Here's how the part is built. I have some questions about the finished solid (model axes, mm). A direction names the side the tool comes from. Coordinates: 2 decimals unless noted, no trailing zeros. Loops run counter-clockwise (first coordinate to the right, second up) from the corner with the lowest first, then second, coordinate; pieces in that order, holes last. Notation, with made-up numbers: M 5.5,33.25 L 38.5,33.25 A13 ccw 38.5,39.25 Z; hole C -27,12 d3. An arc over 180 degrees is marked long. Use CSV: the item, a comma, the result in double quotes. Start each with the question number.
Q1. If we section it at B-B (z = 5.25): Please give me the cut outline in (x, y).
Q2. Please list where these lines run through material, in increasing order: probe 1 along Y at (x, z) = (0, 12.5); probe 2 along Y at (x, z) = (1.5, 10.5). Write a range as [from, to].
Q3. If we section it at C-C (x = 14): Please give me the cut outline in (y, z).
Q4. Which directions (+Z, -Z, +X, -X, +Y, -Y) give clear straight access to the entire face, cutting with the end or side of a thin tool? Please do faces 1 (the flat face through (-14, 0, 18)), 2 (the flat face through (1.204, 14, 19)), 3 (the flat face through (-11, 12, 5.94)), 4 (the flat face through (13, -9, 3)).
Q5. For pin 1 Ø8 at (y, z) = (10, 14.5) entering from +X; pin 2 Ø4 at (x, y) = (-5, 12.5) entering from -Z; pin 3 Ø0.8 at (y, z) = (-14, 19) entering from +X; pin 4 Ø2.5 at (x, z) = (13.5, 2) entering from -Y, each with a flat end and sliding along its axis, tell me the tip position at first contact or that it passes through.
Q6. If we section it at A-A (y = 0): Please give me the cut outline in (x, z), and give its area (3 significant figures).
Q7. If we mould it in two halves opening along X, with no side actions, what happens to faces 5 (the flat face through (0, 14, 18)), 6 (the flat face through (0, -16, 0)), 7 (the flat face through (1.204, -14, 19))? For each: +X half, -X half, draft (parallel to the pull), parting line (faces both ways), or undercut.
Q8. If we section it at D-D (x = 0): Please give me the cut outline in (y, z).
from build123d import *

# Parameters (mm, degrees)
F0_R     = 17
F0_R_2   = 15
F1_DEPTH = 20
F3_DEPTH = 25
F5_DEPTH = 2
F7_DEPTH = 2


with BuildPart() as f1:
    # F0 (on Top) → F1 (new body)
    with BuildSketch(Plane.XY):
        Circle(F0_R)
        Circle(F0_R_2, mode=Mode.SUBTRACT)
    extrude(amount=F1_DEPTH)

    # F2 (on Right) → F3 (cut, symmetric)
    with BuildSketch(Plane.YZ):
        Polygon((-9, 5.94), (-9, -6.120001), (9, -5.76), (9, 5.94), (14, 5.94), (14, 9.000001), (-14, 9.000001), (-14, 5.94), align=None)
    extrude(amount=F3_DEPTH, both=True, mode=Mode.SUBTRACT)

    # F4 (on face) → F5 (join)
    with BuildSketch(Plane.XY.offset(20)):
        with BuildLine():
            ThreePointArc((-14.831288, -2.243409), (-14.998609, -0.204311), (-14.886893, 1.838588))
            Line((-14.886893, 1.838588), (-16.424584, 1.838588))
            Line((-16.424584, 1.838588), (-16.424584, -2.243409))
            Line((-16.424584, -2.243409), (-14.831288, -2.243409))
        make_face()
        with BuildLine():
            Line((-12.919951, -2.243409), (-12.919951, 1.838588))
            Line((-12.919951, 1.838588), (-14.886893, 1.838588))
            ThreePointArc((-14.886893, 1.838588), (-14.998609, -0.204311), (-14.831288, -2.243409))
            Line((-14.831288, -2.243409), (-12.919951, -2.243409))
        make_face()
        with BuildLine():
            Line((14.886893, 1.838588), (12.728207, 1.838588))
            Line((12.728207, 1.838588), (12.728207, -2.243409))
            Line((12.728207, -2.243409), (14.831288, -2.243409))
            ThreePointArc((14.831288, -2.243409), (14.957763, -1.124872), (15, 0))
            ThreePointArc((15, 0), (14.971697, 0.921032), (14.886893, 1.838588))
        make_face()
        with BuildLine():
            Line((16.602479, 1.838588), (14.886893, 1.838588))
            ThreePointArc((14.886893, 1.838588), (14.971697, 0.921032), (15, 0))
            ThreePointArc((15, 0), (14.957763, -1.124872), (14.831288, -2.243409))
            Line((14.831288, -2.243409), (16.602479, -2.243409))
            Line((16.602479, -2.243409), (16.602479, 1.838588))
        make_face()
    extrude(amount=-F5_DEPTH)

    # F6 (on face) → F7 (join)
    with BuildSketch(Plane.XY.offset(20)):
        with BuildLine():
            ThreePointArc((1.204057, 14.951597), (0.034161, 14.999961), (-1.135944, 14.956926))
            Line((-1.135944, 14.956926), (-1.135944, 13.48272))
            Line((-1.135944, 13.48272), (1.204057, 13.48272))
            Line((1.204057, 13.48272), (1.204057, 14.951597))
        make_face()
        with BuildLine():
            Line((1.204057, 16.09272), (-1.135944, 16.09272))
            Line((-1.135944, 16.09272), (-1.135944, 14.956926))
            ThreePointArc((-1.135944, 14.956926), (0.034161, 14.999961), (1.204057, 14.951597))
            Line((1.204057, 14.951597), (1.204057, 16.09272))
        make_face()
        with BuildLine():
            ThreePointArc((1.204057, -14.951597), (0.034161, -14.999961), (-1.135944, -14.956926))
            Line((-1.135944, -14.956926), (-1.135944, -15.857281))
            Line((-1.135944, -15.857281), (1.204057, -15.857281))
            Line((1.204057, -15.857281), (1.204057, -14.951597))
        make_face()
        with BuildLine():
            Line((1.204057, -13.337282), (-1.135944, -13.337282))
            Line((-1.135944, -13.337282), (-1.135944, -14.956926))
            ThreePointArc((-1.135944, -14.956926), (0.034161, -14.999961), (1.204057, -14.951597))
            Line((1.204057, -14.951597), (1.204057, -13.337282))
        make_face()
    extrude(amount=-F7_DEPTH)


solid = f1.part
Results below:
1,outline,"M -14.42,-9 A17 ccw 14.42,-9 L 12,-9 A15 cw -12,-9 Z; M -14.42,9 L -12,9 A15 cw 12,9 L 14.42,9 A17 ccw Z"
2,probe 1,"[-17, -15], [15, 17]"
2,probe 2,"[-16.93, -14.92], [14.92, 16.93]"
3,outline,"M -9.64,0 L -9,0 L -9,5.94 L -9.64,5.94 Z; M -9.64,9 L -5.39,9 L -5.39,20 L -9.64,20 Z; M -2.24,18 L 1.84,18 L 1.84,20 L -2.24,20 Z; M 5.39,9 L 9.64,9 L 9.64,20 L 5.39,20 Z; M 9,0 L 9.64,0 L 9.64,5.94 L 9,5.94 Z"
4,face 1,"-Z"
4,face 2,"+Z, -Z"
4,face 3,"+X, -X"
4,face 4,"-Z, +X, -X"
5,pin 1,"x = 15.91"
5,pin 2,"z = 0"
5,pin 3,"x = 10.2"
5,pin 4,"y = -11.79"
6,outline,"M -17,9 L -15,9 L -15,18 L -12.92,18 L -12.92,20 L -17,20 Z; M 12.73,18 L 15,18 L 15,9 L 17,9 L 17,20 L 12.73,20 Z"
6,area,"52.7 mm^2"
7,face 5,"undercut"
7,face 6,"draft"
7,face 7,"undercut"
8,outline,"M -17,0 L -15,0 L -15,18 L -13.34,18 L -13.34,20 L -17,20 Z; M 13.48,18 L 15,18 L 15,0 L 17,0 L 17,20 L 13.48,20 Z"
